The listing builds one solid part. Answer for the finished solid, in the listing's coordinates (mm). Round coordinates to 2 decimals unless told otherwise and drop trailing zeros. Write each loop counter-clockwise with the first axis right and the second up, starting at its lowest first coordinate (ties: lowest second). Pieces come first, ordered by that corner, then holes. Notation, with made-up numbers: M 42,88.5 L 88,88.5 A23 cw 88,112.5 Z; hole C 64,5.25 d6. An arc over 180 degrees is marked long. Put each result on its own line as item: value. Start each with the question number.
```python
from build123d import *

# Parameters (mm, degrees)
BOSS_EXTRUDE1_DEPTH = 3.175


with BuildPart() as part:
    # Sketch1 → Boss-Extrude1 (new body)
    with BuildSketch(Plane(origin=(0, 0, 0), x_dir=(1, 0, 0), z_dir=(0, 1, 0))):
        with BuildLine():
            Line((-717.55, 504.825), (-717.55, 392.610512242))
            ThreePointArc((-717.55, 392.610512242), (-718.516729937, 387.750432651), (-721.269743879, 383.630256121))
            Line((-721.269743879, 383.630256121), (-761.07006403, 343.82993597))
            ThreePointArc((-761.07006403, 343.82993597), (-761.758317516, 342.799891837), (-762, 341.584871939))
            Line((-762, 341.584871939), (-762, -504.825))
            ThreePointArc((-762, -504.825), (-761.07006403, -507.07006403), (-758.825, -508))
            Line((-758.825, -508), (758.825, -508))
            ThreePointArc((758.825, -508), (761.07006403, -507.07006403), (762, -504.825))
            Line((762, -504.825), (762, 341.584871939))
            ThreePointArc((762, 341.584871939), (761.758317516, 342.799891837), (761.07006403, 343.82993597))
            Line((761.07006403, 343.82993597), (721.269743879, 383.630256121))
            ThreePointArc((721.269743879, 383.630256121), (718.516729937, 387.750432651), (717.55, 392.610512242))
            Line((717.55, 392.610512242), (717.55, 504.825))
            ThreePointArc((717.55, 504.825), (716.62006403, 507.07006403), (714.375, 508))
            Line((714.375, 508), (-714.375, 508))
            ThreePointArc((-714.375, 508), (-716.62006403, 507.07006403), (-717.55, 504.825))
        make_face()
    extrude(amount=BOSS_EXTRUDE1_DEPTH)


solid = part.part
```
Item 1: Flat-ended cylindrical pins translate along their axes: pin 1 (1.6 mm diameter, centred on y = 1, z = -432.5, fed in from +X); pin 2 (1.6 mm diameter, centred on y = 1, z = -458, fed in from -X). Find the tip coordinate at first contact, or state that the pin passes through.
Item 2: Consider line 1 along X through (y, z) = (1.9, -406); line 2 along X through (y, z) = (2.05, -360). Determine where each line is inside the solid, lowest interval first. Write a range as [from, to].
Item 3: Section A-A (z = -440) is taken. Give the vertices of the cut face in (x, y) (3 decimals), and give its area (3 significant figures).
Output values:
1. pin 1: stops at x = 717.55
1. pin 2: stops at x = -717.55
2. line 1: x = [-717.55, 717.55]
2. line 2: x = [-744.9, 744.9]
3. outline: M -717.55,0 L 717.55,0 L 717.55,3.175 L -717.55,3.175 Z
3. area: 4,560 mm^2
